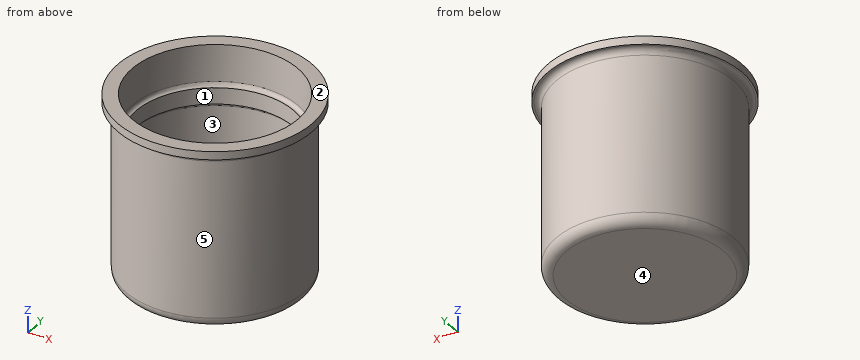
```python
from build123d import *


with BuildPart() as part:
    # Sketch → Revolution (revolve)
    with BuildSketch(Plane.XZ):
        with BuildLine():
            Line((0, 0), (-7.75, 0))
            ThreePointArc((-8.75, 1), (-8.457107, 0.292893), (-7.75, 0))
            Line((-8.75, 1), (-8.75, 16.4))
            ThreePointArc((-8.75, 16.4), (-8.925736, 16.824264), (-9.35, 17))
            Line((-9.35, 17), (-9.55, 17))
            Line((-9.55, 17), (-9.55, 17.8))
            Line((-9.55, 17.8), (-8.15, 17.8))
            Line((-8.15, 17.8), (-8.15, 14.19))
            ThreePointArc((-8.15, 14.19), (-8.035772, 13.914228), (-7.76, 13.8))
            Line((-7.76, 13.8), (-7.75, 13.8))
            Line((-7.75, 13.8), (-7.75, 12.2))
            Line((-7.75, 12.2), (-7.76, 12.2))
            ThreePointArc((-7.76, 12.2), (-8.035772, 12.085772), (-8.15, 11.81))
            Line((-8.15, 11.81), (-8.15, 1.6))
            ThreePointArc((-8.15, 1.6), (-7.857107, 0.892893), (-7.15, 0.6))
            Line((-7.15, 0.6), (0, 0.6))
            Line((0, 0.6), (0, 0))
        make_face()
    revolve(axis=Axis((0, 0, 0), (0, 0, 1)))


solid = part.part
```
CAD build for the part. Positions are in the model's coordinates, mm. Face numbers are marked on the shaded views. A direction names the side the tool comes from. Round coordinates to 2 decimals unless told otherwise and drop trailing zeros. Loops run counter-clockwise (first coordinate to the right, second up) from the corner with the lowest first, then second, coordinate; pieces in that order, holes last. Notation, with made-up numbers: M -24.5,6.5 L -18.5,6.5 A6 cw -18.5,12.5 Z; hole C -11,-10 d11. An arc over 180 degrees is marked long. Use a Markdown table: item, result. Add a question column.
(1) Which spindle directions (+Z, -Z, +X, -X, +Y, -Y) get a long thin tool onto all of the face, cutting with end or side? Do the marked faces 1 and 2. Say none if no direction does.
(2) Flat gauge pins, fed straight in: pin 1 (4.5 mm diameter, centred on x = -0.5, y = 3, fed in from +Z); pin 2 (3 mm diameter, centred on y = 4, z = 6.5, fed in from -X); pin 3 (5 mm diameter, centred on x = 0, z = 12, fed in from +Y). Where does each tip first touch, or does it go through?
(3) Pull direction Z, two halves, no side cores. Call the marked faces 3, 4 and 5: +Z half, -Z half, draft (parallel to the pull), parting line (faces both ways), or undercut.
(4) Cut at C-C (z = 2). Give the cut face in (x, y).
(5) Drill centre lines: line 1 (Y direction, x = 0, z = 7.25); line 2 (Y direction, x = 0, z = 12.8). Where is each one in solid material? Low to high.
Geometry says:
| question | item | result |
|---|---|---|
| 1 | face 1 | +Z |
| 1 | face 2 | +Z, +X, -X, +Y, -Y |
| 2 | pin 1 | stops at z = 0.6 |
| 2 | pin 2 | stops at x = -8.39 |
| 2 | pin 3 | stops at y = 8.75 |
| 3 | face 3 | undercut |
| 3 | face 4 | -Z half |
| 3 | face 5 | draft |
| 4 | outline | C 0,0 d17.5; hole C 0,0 d16.3 |
| 5 | line 1 | y = -8.75 to -8.15, 8.15 to 8.75 |
| 5 | line 2 | y = -8.75 to -7.75, 7.75 to 8.75 |
